```python
from build123d import *

# Parameters (mm, degrees)
CUT_EXTRUDE_1_DEPTH = 2.5
FILLET_1_R          = 0.3
CHAMFER_1_SIZE      = 1


with BuildPart() as part:
    # Эскиз1 → Повернуть1 (revolve)
    with BuildSketch(Plane.XY):
        Polygon((0, 0), (0, 5), (6, 5), (6, 3), (26, 3), (26, 0), align=None)
    revolve(axis=Axis((26, 0, 0), (-1, 0, 0)))

    # Эскиз2 → Вырез-Вытянуть1 (cut)
    with BuildSketch(Plane.ZY):
        Polygon((-1.443375673, 2.5), (-2.886751346, 0), (-1.443375673, -2.5), (1.443375673, -2.5), (2.886751346, 0), (1.443375673, 2.5), align=None)
    extrude(amount=-CUT_EXTRUDE_1_DEPTH, mode=Mode.SUBTRACT)

    # Скругление1
    fillet_1_edges = [part.edges().sort_by_distance(p)[0] for p in [
        (6, -3, 0),
        (0, -5, 0),
    ]]
    fillet(fillet_1_edges, radius=FILLET_1_R)

    # Фаска1
    chamfer_1_edges = [part.edges().sort_by_distance(p)[0] for p in [
        (26, -3, 0),
    ]]
    chamfer(chamfer_1_edges, length=CHAMFER_1_SIZE)


solid = part.part
```
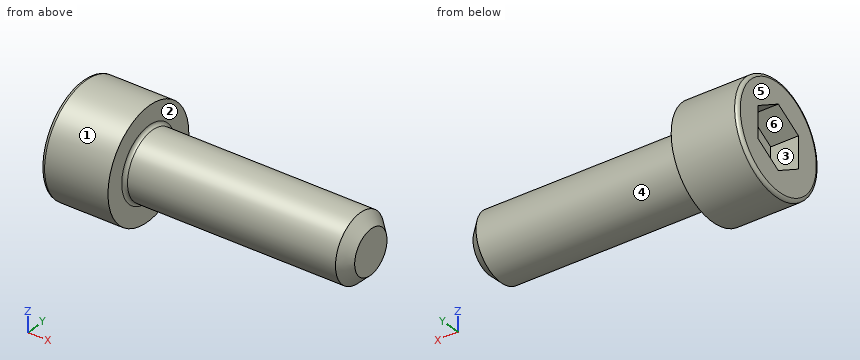
Geometry: final body of the model. Coordinates: model frame, mm. Face numbers are marked on the shaded views. A direction names the side the tool comes from. Round coordinates to 2 decimals unless told otherwise and drop trailing zeros. Loops run counter-clockwise (first coordinate to the right, second up) from the corner with the lowest first, then second, coordinate; pieces in that order, holes last. Notation, with made-up numbers: (22.5, -29.5) -> (37.5, -29.5) arc R20 cw to (37.5, -1.5) -> close; hole circle Ø11 at (-10.75, 27.25). An arc over 180 degrees is marked (long way). Write each question's results on one line, items separated by ' | '.
Item 1: Cut plane A-A on z = 0. Return the cut outline in (x, y).
Answers below:
outline: (0, -4.7) arc R0.3 ccw to (0.3, -5) -> (6, -5) -> (6, -3.3) arc R0.3 cw to (6.3, -3) -> (25, -3) -> (26, -2) -> (26, 2) -> (25, 3) -> (6.3, 3) arc R0.3 cw to (6, 3.3) -> (6, 5) -> (0.3, 5) arc R0.3 ccw to (0, 4.7) -> (0, 2.5) -> (2.5, 2.5) -> (2.5, -2.5) -> (0, -2.5) -> close
Item 2: Set-up query: the marked faces 4, 5 and 6. Return all of +Z, -Z, +X, -X, +Y, -Y with unobstructed straight access to the full face (end or side cutting, diameter ignored); none if empty.
Answers below:
face 4: +X | face 5: +Z, -Z, -X, +Y, -Y | face 6: -X
Item 3: Cut plane C-C on x = 3.5. Return the cut outline in (y, z).
Answers below:
outline: circle Ø10 at (0, 0)
Item 4: Pin query (flat end, axial travel): pin 1 Ø6 at (x, y) = (4, 3.5) entering from +Z; pin 2 Ø2 at (x, y) = (21.5, -3.5) entering from +Z; pin 3 Ø1 at (x, z) = (4.5, 2.5) entering from +Y. Return the tip coordinate at first contact, or that it passes through.
Answers below:
pin 1: stops at z = 4.97 | pin 2: stops at z = 1.66 | pin 3: stops at y = 4.58
Item 5: Pull-direction query (Y, two-part tool) for the marked faces 1, 2 and 3; classes: pulls with the +Y half, pulls with the -Y half, needs draft (parallel to the pull), parting line crosses it, or undercut.
Answers below:
face 1: parting line crosses it | face 2: needs draft | face 3: undercut
Item 6: Line query: probe 1 along X at (y, z) = (0.25, 4.25); probe 2 along Y at (x, z) = (20, 0). Output: solid intervals per line, ascending. Write a range as [from, to].
Answers below:
probe 1: x = [0, 6] | probe 2: y = [-3, 3]
Item 7: Cut plane B-B on x = 13.75. Return the cut outline in (y, z).
Answers below:
outline: circle Ø6 at (0, 0)
